Read the model definition and answer for the solid it produces. Units are mm, in the model's axes. Face numbers are marked on the shaded views. A direction names the side the tool comes from. Give positions to 0.01 mm unless a question says otherwise; leave off trailing zeros. Order: outer loops, then holes, each group sorted by start corner. A loop starts at its lowest first (then second) coordinate and runs counter-clockwise, first axis right, second up. Notation, with made-up numbers: M 47,-18 L 92,-18 A14 ccw 92,-12 Z; hole C 0.5,82.5 d7. An arc over 180 degrees is marked long. Write item = value, one per line. Start each with the question number.
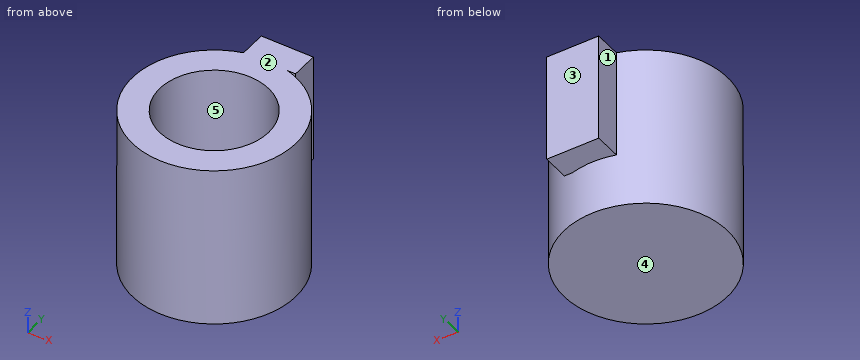
from build123d import *

# Parameters (mm, degrees)
F0_R     = 38.1
F1_DEPTH = 76.2
F2_R     = 25.4
F3_DEPTH = 50.8
F4_W     = 24.265683
F4_H     = 12.642243
F5_DEPTH = 50.8


with BuildPart() as f1:
    # F0 (on Top) → F1 (new body)
    with BuildSketch(Plane.XY):
        Circle(F0_R)
    extrude(amount=F1_DEPTH)

    # F2 (on face) → F3 (cut)
    with BuildSketch(Plane.XY.offset(76.2)):
        Circle(F2_R)
    extrude(amount=-F3_DEPTH, mode=Mode.SUBTRACT)

    # F4 (on face) → F5 (join)
    with BuildSketch(Plane.XY.offset(76.2)):
        with Locations((1.853868, 43.008349)):
            Rectangle(F4_W, F4_H)
    extrude(amount=-F5_DEPTH)


solid = f1.part
1) Find section D-D on z = 7. Determine the outline of the cut face in (x, y), plus the area to 3 significant figures.
2) For a pull along Y with two mould halves and no side action, classify the marked faces 3, 4 and 5 as pulls with the +Y half, pulls with the -Y half, needs draft (parallel to the pull), parting line crosses it, or undercut.
3) Find section A-A on z = 27. Determine the outline of the cut face in (x, y), plus the area to 3 significant figures.
4) Find section C-C on x = 0. Determine the outline of the cut face in (y, z).
5) Find the intervals of material crossed by probe 1 along Y at (x, z) = (0, 47); probe 2 along X at (y, z) = (11, 55); probe 3 along Y at (x, z) = (18, 54.5), in increasing order. Write a range as [from, to].
6) For the marked faces 1 and 2, determine the directions among +Z, -Z, +X, -X, +Y, -Y from which every point of the face is accessible in a straight line to the end or side of a thin tool.
7) Find section B-B on y = -2.5. Determine the outline of the cut face in (x, z), plus the area to 3 significant figures.
8) Each of these flat-tipped pins is pushed along its axis until it touches: P1, Ø1.1, axis at x = 12.5, z = 54, coming from the -Y side; P2, Ø6.5, axis at x = 3.5, y = 43, coming from the -Z side; P3, Ø6.5, axis at y = 42.5, z = 44, coming from the -X side. Where does it stop, or does it pass through?
Numbers:
q1.outline = C 0,0 d76.2
q1.area = 4,560 mm2
q2.face_3 = pulls with the +Y half
q2.face_4 = needs draft
q2.face_5 = undercut
q3.outline = M -10.28,36.69 A38.1 ccw long 10.28,36.69 L 13.99,36.69 L 13.99,49.33 L -10.28,49.33 Z; hole C 0,0 d50.8
q3.area = 2,820 mm2
q4.outline = M -38.1,0 L 38.1,0 L 38.1,25.4 L 49.33,25.4 L 49.33,76.2 L 25.4,76.2 L 25.4,25.4 L -25.4,25.4 L -25.4,76.2 L -38.1,76.2 Z
q5.probe_1 = [-38.1, -25.4], [25.4, 49.33]
q5.probe_2 = [-36.48, -22.89], [22.89, 36.48]
q5.probe_3 = [-33.58, -17.92], [17.92, 33.58]
q6.face_1 = +Z, -Z, -X, +Y
q6.face_2 = +Z, +X, -X, +Y, -Y
q7.outline = M -38.02,0 L 38.02,0 L 38.02,76.2 L 25.28,76.2 L 25.28,25.4 L -25.28,25.4 L -25.28,76.2 L -38.02,76.2 Z
q7.area = 3,230 mm2
q8.P1 = -36.18
q8.P2 = 25.4
q8.P3 = -10.28
